Study the drawing (mm; zero at the part's minimum x, y, z) and answer. A direction names the side the tool comes from. Give positions to 0.01 mm unless a question says otherwise; leave off trailing zeros. Order: outer loops, then holes, each group sorted by start corner. A loop starts at its lowest first (then second) coordinate and runs counter-clockwise, first axis right, second up. Notation, with made-up numbers: (28, -6) - (47, -6) arc R29 ccw to (47, 29) - close; hole circle Ø3 at (-11, 31.5). An arc over 180 degrees is marked (long way). Return JSON: item names as keys, results as strings.
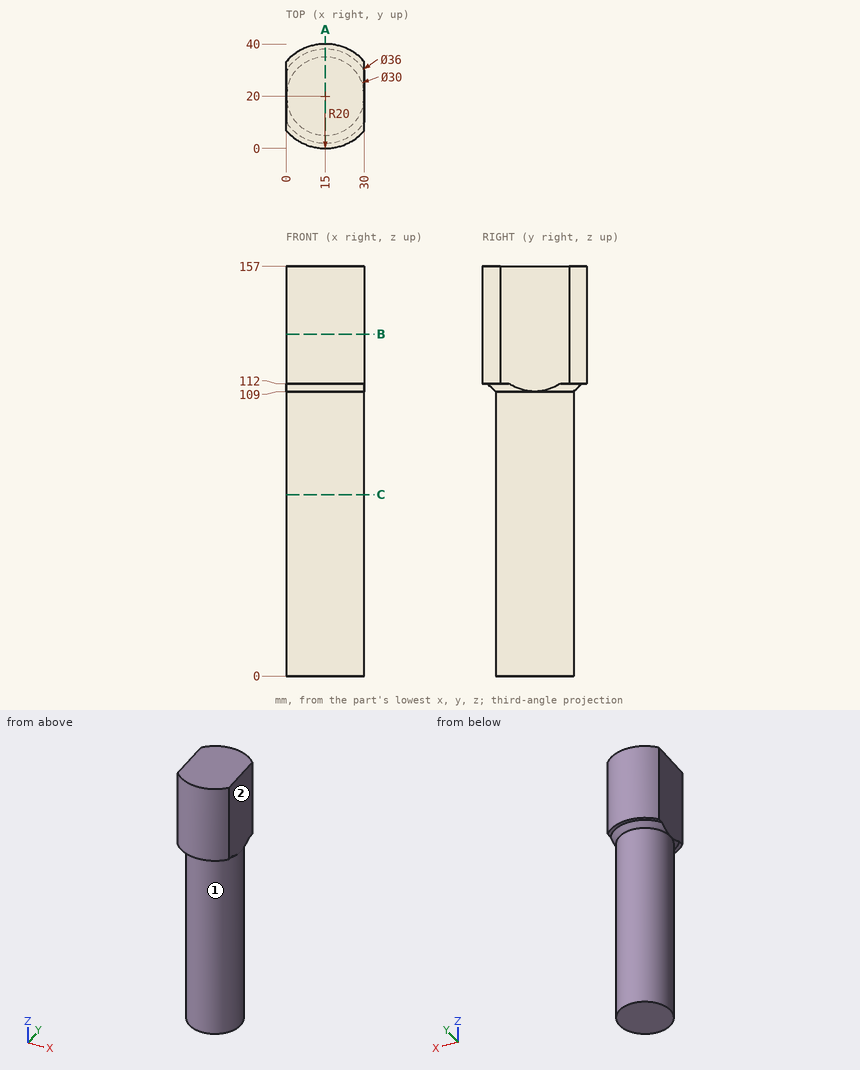
Q1. Consider L1, parallel to Y at x = 6.5, z = 87; L2, parallel to X at y = 34, z = 113; L3, parallel to Y at x = 19.5, z = 131. Determine where each line is inside the solid, lowest interval first.
Values:
{"L1": "y = 7.64 to 32.36", "L2": "x = 0.72 to 29.28", "L3": "y = 0.51 to 39.49"}
Q2. For the marked faces 1 and 2, determine the directions among +Z, -Z, +X, -X, +Y, -Y from which every point of the face is accessible in a straight line to the end or side of a thin tool.
Values:
{"face 1": "-Z", "face 2": "+Z, -Z, +X, +Y, -Y"}
Q3. A cutting plane is placed at A-A (x = 15). Write down the section's boundary in (y, z).
Values:
{"outline": "(0, 112) - (2, 112) - (5, 109) - (5, 0) - (35, 0) - (35, 109) - (38, 112) - (40, 112) - (40, 157) - (0, 157) - close"}
Q4. Given pin 1 (1.5 mm diameter, centred on y = 29, z = 34, fed in from -X); pin 2 (3 mm diameter, centred on x = 16, y = 2.5, fed in from -Z); pin 3 (12 mm diameter, centred on x = 24, z = 62, fed in from -Y), each flat-ended and moving along its own axis, determine where each tip first touches the part or whether it passes through.
Values:
{"pin 1": "stops at x = 2.47", "pin 2": "stops at z = 110.03", "pin 3": "stops at y = 5.3"}
Q5. A cutting plane is placed at C-C (z = 69.5). Write down the section's boundary in (x, y), and give its area (3 significant figures).
Values:
{"outline": "circle Ø30 at (15, 20)", "area": "707 mm²"}
Q6. A cutting plane is placed at B-B (z = 131). Write down the section's boundary in (x, y), and give its area (3 significant figures).
Values:
{"outline": "(0, 6.77) arc R20 ccw to (30, 6.77) - (30, 33.23) arc R20 ccw to (0, 33.23) - close", "area": "1,080 mm²"}
